from build123d import *

# Parameters (mm, degrees)
F0_W     = 83.305214
F0_H     = 60.44998
F1_DEPTH = 76.2


with BuildPart() as f1:
    # F0 (on Front) → F1 (new body)
    with BuildSketch(Plane.XZ):
        Rectangle(F0_W, F0_H)
        Polygon((10.742642, 18.606802), (21.485284, 0), (10.742642, -18.606802), (-10.742642, -18.606802), (-21.485284, 0), (-10.742642, 18.606802), align=None, mode=Mode.SUBTRACT)
    extrude(amount=F1_DEPTH)


solid = f1.part
Input: part model. Units: mm. Frame: model coordinates. A direction names the side the tool comes from. Round coordinates to 2 decimals unless told otherwise and drop trailing zeros. Order: outer loops, then holes, each group sorted by start corner. A loop starts at its lowest first (then second) coordinate and runs counter-clockwise, first axis right, second up. Notation, with made-up numbers: (-12.5, 85.5) - (-3.5, 85.5) arc R22 cw to (-3.5, 103.5) - close; hole circle Ø11 at (-39.75, 8.25). An arc over 180 degrees is marked (long way). Use a Markdown table: item, result.
1. Access query for faces 1 (the face through (18, 0, 7)), 2 (the face through (-16.04, -37.57, -9.43)). Directions: +Z, -Z, +X, -X, +Y, -Y. A direction counts if a zero-diameter tool reaches every point of the face in a straight line with its end or side. Return the directions, or none.
Evaluation:
| item | result |
|---|---|
| face 1 | +Z, -Z, +X, -X, +Y |
| face 2 | +Y, -Y |
2. Mould query, pull axis X, two halves, no side actions, for faces 3 (the face through (-1, -38, -30.225)), 4 (the face through (16.04, -37.57, 9.43)), 5 (the face through (0, -38, -18.607)), 6 (the face through (41.653, -38, 0)). Classes: +X half, -X half, draft (parallel to the pull), parting line (faces both ways), or undercut.
Evaluation:
| item | result |
|---|---|
| face 3 | draft |
| face 4 | undercut |
| face 5 | undercut |
| face 6 | +X half |
3. Section B-B on y = -45. Return the cut outline in (x, z) (3 decimals), then the cut area to 3 significant figures.
Evaluation:
| item | result |
|---|---|
| outline | (-41.653, -30.225) - (41.653, -30.225) - (41.653, 30.225) - (-41.653, 30.225) - close; hole (-21.485, 0) - (-10.743, -18.607) - (10.743, -18.607) - (21.485, 0) - (10.743, 18.607) - (-10.743, 18.607) - close |
| area | 3,840 mm^2 |
4. Section A-A on x = 0. Return the cut outline in (y, z), then the cut area to 3 significant figures.
Evaluation:
| item | result |
|---|---|
| outline | (-76.2, -30.22) - (0, -30.22) - (0, -18.61) - (-76.2, -18.61) - close; (-76.2, 18.61) - (0, 18.61) - (0, 30.22) - (-76.2, 30.22) - close |
| area | 1,770 mm^2 |
5. Section C-C on z = 11. Return the cut outline in (x, y).
Evaluation:
| item | result |
|---|---|
| outline | (-41.65, -76.2) - (-15.13, -76.2) - (-15.13, 0) - (-41.65, 0) - close; (15.13, -76.2) - (41.65, -76.2) - (41.65, 0) - (15.13, 0) - close |
6. Material intervals for probe 1 along Z at (x, y) = (-3.5, -61.5); probe 2 along X at (y, z) = (-49, -17); probe 3 along X at (y, z) = (-67, -6.5), sorted ascending.
Evaluation:
| item | result |
|---|---|
| probe 1 | -30.22 to -18.61, 18.61 to 30.22 |
| probe 2 | -41.65 to -11.67, 11.67 to 41.65 |
| probe 3 | -41.65 to -17.73, 17.73 to 41.65 |
